Source: CAD feature listing. Evaluate the final solid. Frame: model axes, mm. Face numbers are marked on the shaded views. A direction names the side the tool comes from. Round coordinates to 2 decimals unless told otherwise and drop trailing zeros. Write each loop counter-clockwise with the first axis right and the second up, starting at its lowest first coordinate (ties: lowest second). Pieces come first, ordered by that corner, then holes. Notation, with made-up numbers: M 85,83 L 93,83 A18 cw 93,108 Z; hole C -21.75,84.25 d11. An arc over 180 degrees is marked long. Use a Markdown table: item, result.
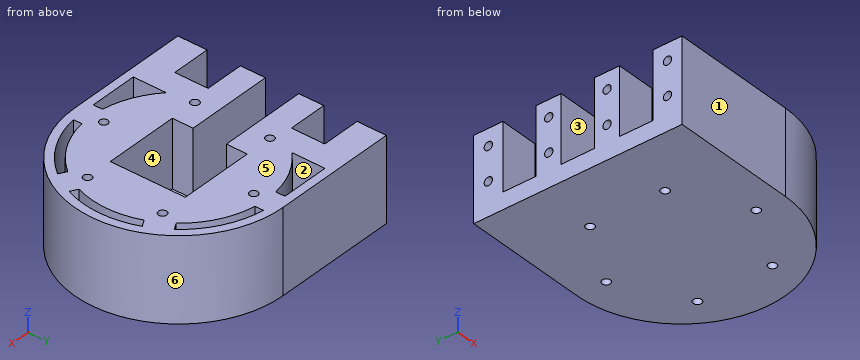
Autodesk Inventor part; units mm, degrees
ref_plane "YZ Plane" through (0, 0, 0) normal (1, 0, 0) x (0, 1, 0)
ref_plane "XZ Plane" through (0, 0, 0) normal (0, 1, 0) x (-1, 0, 0)
ref_plane "XY Plane" through (0, 0, 0) normal (0, 0, 1) x (1, 0, 0)
sketch "Sketch1" plane through (0, 0, 0) normal (0, 0, 1) x (1, 0, 0)
  circle A0 centre (0, 0) radius 62.5 construction
  line L0 (0, 62.5) -> (-75, 62.5)
  line L1 (-75, 62.5) -> (-75, -62.5)
  line L2 (-75, -62.5) -> (0, -62.5)
  arc A1 (0, -62.5) -> (0, 62.5) centre (0, 0) ccw
  dimension "d0" = 125
  dimension "d1" = 75
  dimension "d2" = 75
extrude "Extrusion1" add sketch "Sketch1" along normal blind 50
sketch "Sketch6" plane through (0, 0, 50) normal (0, 0, 1) x (1, 0, 0)
  line L0 (-22.5, -22.5) -> (22.5, -22.5)
  line L1 (22.5, -22.5) -> (22.5, 22.5)
  line L2 (22.5, 22.5) -> (-22.5, 22.5)
  line L3 (-22.5, 22.5) -> (-22.5, -22.5)
  line L4 (-22.5, -22.5) -> (22.5, 22.5) construction
  line L5 (22.5, -22.5) -> (-22.5, 22.5) construction
  point P0 (0, 0)
  dimension "d23" = 45
  dimension "d24" = 45
extrude "Extrusion6" cut sketch "Sketch6" against normal blind 40
sketch "Sketch7" plane through (-22.5, -22.5, 50) normal (1, 0, 0) x (0, 0, -1)
  line L0 (40, 32.5) -> (0, 32.5)
  line L1 (0, 32.5) -> (0, 12.5)
  line L2 (0, 12.5) -> (40, 12.5)
  line L3 (40, 12.5) -> (40, 32.5)
  point P0 (50, 22.5)
  point P1 (40, 22.5)
  dimension "d27" = 40
  dimension "d28" = 20
  dimension "d29" = 10
extrude "Extrusion7" cut sketch "Sketch7" against normal through all
sketch "Sketch9" plane through (0, 0, 50) normal (0, 0, 1) x (1, 0, 0)
  circle A0 centre (0, 45) radius 2.5
  circle A1 centre (-38.9711, 22.5) radius 2.5
  circle A2 centre (-38.9711, -22.5) radius 2.5
  circle A3 centre (0, -45) radius 2.5
  circle A4 centre (38.9711, -22.5) radius 2.5
  circle A5 centre (38.9711, 22.5) radius 2.5
  point P0 (0, 0)
  dimension "d35" = 5
  dimension "d36" = 45
  dimension "d39" = 360
extrude "Extrusion9" cut sketch "Sketch9" against normal through all
sketch "Sketch10" plane through (0, 0, 50) normal (0, 0, 1) x (1, 0, 0)
  circle A0 centre (0, 0) radius 52.5
  arc A1 (0, -57.5) -> (0, -57.5) centre (0, 0) ccw
  line L0 (0, -57.5) -> (-75, -57.5)
  line L1 (-75, 57.5) -> (-75, -57.5)
  line L2 (0, -57.5) -> (-75, -57.5)
  line L3 (0, 57.5) -> (-75, 57.5)
  circle A2 centre (0, 0) radius 57.5 construction
  arc A3 (0, -57.5) -> (0, 57.5) centre (0, 0) ccw
  line L4 (-75, -10) -> (-75, 10)
  point P0 (-75, 0)
  dimension "d111" = 115
  dimension "d43" = 105
  dimension "d114" = 90
extrude "Extrusion10" cut sketch "Sketch10" against normal blind 40
sketch "Sketch12" plane through (0, 0, 10) normal (0, 0, 1) x (1, 0, 0)
  line L0 (0, 0) -> (77.9423, -45) construction
  line L1 (0, 0) -> (90, 0) construction
  line L2 (48.75, -19.4856) -> (57.4855, -24.529)
  line L3 (41.25, -32.476) -> (49.9855, -37.5194)
  arc A0 (41.25, -32.476) -> (48.75, -19.4856) centre (0, 0) ccw
  arc A1 (49.9877, -37.5164) -> (57.484, -24.5324) centre (-4.3593, 2.5168) ccw
  line L4 (41.25, 32.476) -> (49.9855, 37.5194)
  arc A2 (48.75, 19.4856) -> (41.25, 32.476) centre (0, 0) ccw
  line L5 (48.75, 19.4856) -> (57.4855, 24.529)
  arc A3 (57.4855, 24.529) -> (49.9855, 37.5194) centre (-4.3593, -2.5168) ccw
  line L6 (0, 0) -> (0, -109.4234) construction
  line L7 (7.5, -51.9615) -> (7.5, -62.0484)
  line L8 (-7.5, -51.9615) -> (-7.5, -62.5)
  line L9 (0, -62.5) -> (-7.5, -62.5)
  arc A4 (-7.5, -51.9615) -> (7.5, -51.9615) centre (0, 0) ccw
  line L10 (-7.5, 51.9615) -> (-7.5, 62.5)
  line L11 (0, 62.5) -> (-7.5, 62.5)
  arc A5 (7.5, 51.9615) -> (-7.5, 51.9615) centre (0, 0) ccw
  arc A6 (-51.5388, -10) -> (-51.5388, 10) centre (0, 0) ccw
  arc A7 (0, -62.5) -> (0, 62.5) centre (0, 0) ccw
  line L12 (-75, -62.5) -> (0, -62.5) construction
  arc A8 (0, -62.5) -> (7.5, -62.0484) centre (0, 0) ccw
  line L13 (7.5, 51.9615) -> (7.5, 62.0484)
  arc A9 (7.5, 62.0484) -> (0, 62.5) centre (0, 0) ccw
  point P0 (54.0974, -31.2332)
  dimension "d50" = 30
  dimension "d52" = 15
  dimension "d53" = 52.5
  dimension "d54" = 67.5
  dimension "d57" = 60
  dimension "d61" = 15
extrude "Extrusion11" add sketch "Sketch12" along normal blind 40 contours L2 A7 A1 L3 A0 | A2 L4 A3 L5 | A7 A1 | A3 A7 | L7 A7 L9 L8 A4 | A5 L10 L11 A7 L13
sketch "Sketch16" plane through (0, 0, 10) normal (0, 0, 1) x (1, 0, 0)
  line L0 (-22.5, 10) -> (-51.5388, 10)
  line L1 (-51.5388, 10) -> (-51.5388, 62.5)
  line L2 (-36.5388, 62.5) -> (-36.5388, 37.6983)
  arc A0 (-36.5388, 37.6983) -> (-51.5388, 10) centre (0, 0) ccw
  arc A1 (-7.5, 51.9615) -> (-51.5388, 10) centre (0, 0) ccw
  line L3 (-36.5388, 62.5) -> (-51.5388, 62.5)
  line L4 (0, 0) -> (-111.9606, 0) construction
  line L5 (-51.5388, -10) -> (-51.5388, -62.5)
  line L6 (-36.5388, -62.5) -> (-36.5388, -37.6983)
  arc A2 (-51.5388, -10) -> (-36.5388, -37.6983) centre (0, 0) ccw
  line L7 (-36.5388, -62.5) -> (-51.5388, -62.5)
  point P0 (-44.0388, -62.5)
  dimension "d69" = 15
extrude "Extrusion14" add sketch "Sketch16" along normal blind 40
sketch "Sketch17" plane through (0, 0, 10) normal (0, 0, 1) x (1, 0, 0)
  line L0 (-51.5388, 57.5) -> (-51.5388, 10)
  line L1 (-51.5388, 10) -> (-75, 10)
  line L2 (-75, -57.5) -> (-75, 57.5)
  line L3 (-51.5388, 25) -> (-75, 25)
  line L4 (-51.5388, -10) -> (-51.5388, -57.5)
  line L5 (-51.5388, -10) -> (-75, -10)
  line L6 (-51.5388, -25) -> (-75, -25)
  line L7 (-51.5388, 25) -> (-51.5388, 10)
  line L8 (-75, 25) -> (-75, 10)
  line L9 (-75, -10) -> (-75, -25)
  line L10 (-51.5388, -10) -> (-51.5388, -25)
  point P0 (0, 0)
  point P1 (-51.5388, 67.5)
  point P2 (-75, -67.5)
  point P3 (-75, 67.5)
  point P4 (-51.5388, -67.5)
  point P5 (-75, -62.5)
  point P6 (-75, 62.5)
  point P7 (-51.5388, 62.5)
  point P8 (-51.5388, -62.5)
  dimension "d72" = 15
  dimension "d73" = 15
extrude "Extrusion15" add sketch "Sketch17" along normal blind 40
sketch "Sketch19" plane through (0, 0, 10) normal (0, 0, 1) x (1, 0, 0)
  line L0 (-75, 62.5) -> (-51.5388, 62.5)
  line L1 (-75, 25) -> (-75, -25)
  line L2 (-51.5388, 62.5) -> (-75, 62.5)
  line L3 (-75, 62.5) -> (-75, 45)
  line L4 (-75, 45) -> (-51.5388, 45)
  line L5 (-51.5388, 45) -> (-51.5388, 62.5)
  line L6 (-51.5388, -62.5) -> (-75, -62.5)
  line L7 (-75, 62.5) -> (-75, -62.5)
  line L8 (-51.5388, -62.5) -> (-75, -62.5)
  line L9 (-75, -62.5) -> (-75, -45)
  line L10 (-75, -45) -> (-51.5388, -45)
  line L11 (-51.5388, -45) -> (-51.5388, -62.5)
  point P0 (0, 0)
  dimension "d84" = 17.5
  dimension "d85" = 17.5
extrude "Extrusion16" add sketch "Sketch19" along normal blind 40
sketch "Sketch18" plane through (-75, -62.5, 0) normal (-1, 0, 0) x (0, 0, 1)
  circle A0 centre (40, 45) radius 2.5
  circle A1 centre (20, 45) radius 2.5
  line L0 (50, 52.5) -> (50, 37.5)
  line L1 (0, 125) -> (0, 0)
  circle A2 centre (40, 80) radius 2.5
  circle A3 centre (20, 80) radius 2.5
  circle A4 centre (20, 116.25) radius 2.5
  circle A5 centre (20, 8.75) radius 2.5
  circle A6 centre (40, 8.75) radius 2.5
  circle A7 centre (40, 116.25) radius 2.5
  line L2 (0, 125) -> (50, 125)
  line L3 (10, 87.5) -> (50, 87.5)
  line L4 (10, 52.5) -> (50, 52.5)
  line L5 (0, 0) -> (50, 0)
  point P0 (0, 62.5)
  dimension "d76" = 5
  dimension "d77" = 5
  dimension "d78" = 10
  dimension "d80" = 20
  dimension "d91" = 5
  dimension "d92" = 5
  dimension "d94" = 5
  dimension "d95" = 5
  dimension "d96" = 5
  dimension "d97" = 5
  dimension "d115" = 8.75
  dimension "d116" = 7.5
  dimension "d117" = 7.5
  dimension "d118" = 8.75
extrude "Extrusion18" cut sketch "Sketch18" against normal blind 25
properties part number "SJ001" material "ABS Plastic"
Q1. Reachability of the marked faces 1, 2 and 3 from +Z, -Z, +X, -X, +Y, -Y: full face, straight path, thin tool, end or side. Return the list, or none.
Results are:
| item | result |
|---|---|
| face 1 | +Z, -Z, +X, -X, -Y |
| face 2 | +Z |
| face 3 | +Z, -X |
Q2. Section C-C on x = -28.5. Return loops of the section in (y, z).
Results are:
| item | result |
|---|---|
| outline | M -62.5,0 L 62.5,0 L 62.5,50 L 57.5,50 L 57.5,10 L 44.09,10 L 44.09,50 L 10,50 L 10,10 L -10,10 L -10,50 L -44.09,50 L -44.09,10 L -57.5,10 L -57.5,50 L -62.5,50 Z |
Q3. Section A-A on z = 4.5. Return loops of the section in (x, y), plus the area to 3 significant figures.
Results are:
| item | result |
|---|---|
| outline | M -75,-62.5 L 0,-62.5 A62.5 ccw 0,62.5 L -75,62.5 Z; hole C -38.97,-22.5 d5; hole C -38.97,22.5 d5; hole C 0,-45 d5; hole C 0,45 d5; hole C 38.97,-22.5 d5; hole C 38.97,22.5 d5 |
| area | 15,400 mm^2 |
Q4. Line query: L1, parallel to Y at x = -69, z = 31.5; L2, parallel to Z at x = -63, y = 54; L3, parallel to Y at x = 0, z = 32. Output: solid intervals per line, ascending.
Results are:
| item | result |
|---|---|
| L1 | -62.5 to -45, -25 to -10, 10 to 25, 45 to 62.5 |
| L2 | 0 to 17.51, 22.49 to 37.51, 42.49 to 50 |
| L3 | -62.5 to -47.5, -42.5 to -22.5, 22.5 to 42.5, 47.5 to 62.5 |
Q5. Mould query, pull axis X, two halves, no side actions, for the marked faces 4, 5 and 6. Classes: +X half, -X half, draft (parallel to the pull), parting line (faces both ways), or undercut.
Results are:
| item | result |
|---|---|
| face 4 | undercut |
| face 5 | draft |
| face 6 | +X half |
Q6. Section D-D on z = 19.5. Give the number of separate pieces and of enclosed holes in the cut face, plus the area to 3 significant figures.
Results are:
| item | result |
|---|---|
| separate pieces | 1 |
| enclosed holes | 11 |
| area | 9,630 mm^2 |
Q7. First-contact query: pin 1 Ø4.5 at (y, z) = (17.5, 40) entering from -X; pin 2 Ø10 at (x, z) = (23.5, 20) entering from -Y; pin 3 Ø12 at (x, z) = (36, 16.5) entering from +Y; pin 4 Ø22 at (x, y) = (-25, 51.5) entering from +Z. Flat tips, straight axial feed; report the tip coordinate or a pass-through.
Results are:
| item | result |
|---|---|
| pin 1 | x = -50 |
| pin 2 | y = -59.7 |
| pin 3 | y = 54.83 |
| pin 4 | z = 50 |
Q8. Section B-B on y = 0. Return loops of the section in (x, z).
Results are:
| item | result |
|---|---|
| outline | M -75,0 L 62.5,0 L 62.5,50 L 57.5,50 L 57.5,10 L 52.5,10 L 52.5,50 L 22.5,50 L 22.5,10 L -75,10 Z |
